Design review of the part built by this model. Coordinates are the model's own, in mm. A direction names the side the tool comes from. Round coordinates to 2 decimals unless told otherwise and drop trailing zeros. Write each loop counter-clockwise with the first axis right and the second up, starting at its lowest first coordinate (ties: lowest second). Pieces come first, ordered by that corner, then holes. Notation, with made-up numbers: (89, 9.25) -> (130, 9.25) arc R13 cw to (130, 34.25) -> close; hole circle Ø6 at (69.5, -21). An arc over 180 degrees is marked (long way). One line per question, with ' | ' between items. Start each with the question number.
1) For faces 1 (the flat face through (30, -9, 261.14)), 2 (the flat face through (101.7, -9.39, 180.89)), 3 (the flat face through (-151.499, -9, -110)), list the 3-axis set-ups (+Z, -Z, +X, -X, +Y, -Y) from which the entire face can be reached by the end or side of a thin tool; tool diameter is ignored.
2) Insertion check: pin 1 Ø1.5 at (x, y) = (-53, -9) entering from -Z. The pin has a flat end and moves straight along its axis. Give the tip position at first contact, or say it passes through.
3) Mouldability with a two-part tool opening along Z and no side actions: class faces 4 (the flat face through (204.101, -9, -110)), 5 (the flat face through (110.6, -9.39, 206.21)), 6 (the flat face through (24, -9, -100.81)) as +Z half, -Z half, draft (parallel to the pull), parting line (faces both ways), or undercut.
4) For probe 1 along X at (y, z) = (-16.75, 207); probe 2 along Z at (x, y) = (-53.5, -5.25); probe 3 along X at (y, z) = (-16, 201.5), list the stretches that pass through material, from the lowest coordinate up.
5) Consider section B-B (x = 83). Give the boundary of the cut face in (y, z), then the cut area to 3 significant figures.
6) Consider section A-A (y = -15.75). Give the boundary of the cut face in (x, z).
```python
from build123d import *

# Parameters (mm, degrees)
F0_W     = 76.2
F0_H     = 19.05
F1_DEPTH = 19.05


with BuildPart() as f1:
    # F0 (on Front) → F1 (new body)
    with BuildSketch(Plane.XZ):
        Polygon((280.301026, 261.140416), (-227.698974, 261.140416), (-227.698974, -100.809584), (-151.498974, -100.809584), (204.101026, -100.809584), (280.301026, -100.809584), align=None)
        Polygon((-74.679661, -11.017117), (-60.185768, -23.379542), (-93.152235, -62.029924), (-107.646129, -49.667499), align=None, mode=Mode.SUBTRACT)
        Polygon((94.351287, 187.157308), (127.317754, 225.80769), (141.811647, 213.445264), (108.84518, 174.794882), align=None, mode=Mode.SUBTRACT)
        with Locations((-189.598974, -110.334584)):
            Rectangle(F0_W, F0_H)
        with Locations((242.201026, -110.334584)):
            Rectangle(F0_W, F0_H)
    extrude(amount=F1_DEPTH)


solid = f1.part
```
From the geometry:
1) face 1: +Z, +X, -X, +Y, -Y | face 2: +Y, -Y | face 3: -Z, +Y, -Y
2) pin 1: stops at z = -100.81
3) face 4: draft | face 5: undercut | face 6: -Z half
4) probe 1: x = -227.7 to 111.28, 136.31 to 280.3 | probe 2: z = -100.81 to 261.14 | probe 3: x = -227.7 to 106.58, 131.62 to 280.3
5) outline: (-19.05, -100.81) -> (0, -100.81) -> (0, 261.14) -> (-19.05, 261.14) -> close | area: 6,900 mm2
6) outline: (-227.7, -119.86) -> (-151.5, -119.86) -> (-151.5, -100.81) -> (204.1, -100.81) -> (204.1, -119.86) -> (280.3, -119.86) -> (280.3, 261.14) -> (-227.7, 261.14) -> close; hole (-107.65, -49.67) -> (-93.15, -62.03) -> (-60.19, -23.38) -> (-74.68, -11.02) -> close; hole (94.35, 187.16) -> (108.85, 174.79) -> (141.81, 213.45) -> (127.32, 225.81) -> close
